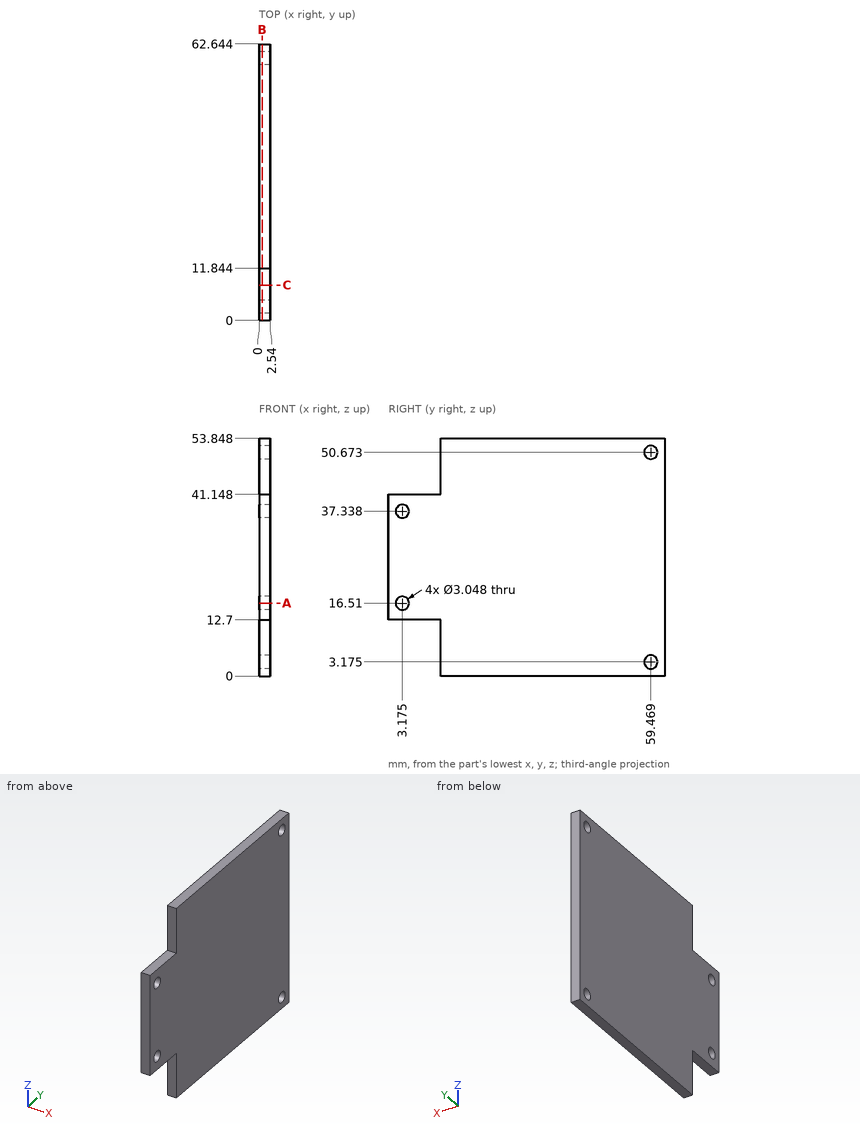
Geometry check sheet. Reference: drawing and pictorial views, mm from the part's lowest x, y, z. Coordinates: 2 decimals unless noted, no trailing zeros. Order: outer loops, then holes, each group sorted by start corner. A loop starts at its lowest first (then second) coordinate and runs counter-clockwise, first axis right, second up.
Item 1: Section check C-C (y = 8). Enter the section's corners in (x, z).
Item 2: Section check B-B (x = 0.65). Enter the section's corners in (y, z) (1 decimal).
Item 3: Section check A-A (z = 16.51). Enter the section's corners in (x, y), plus the area to 3 significant figures.
Item 4: Scan lines: line 1 along Y through (x, z) = (0.6, 50.5) (1 decimal); line 2 along Y through (x, z) = (1.1, 42.5); line 3 along Y through (x, z) = (0.3, 17.5). Record each from-to range of solid material in increasing order.
Item 5: Depth check by flat-ended pin: pin 1 (1.3 mm diameter, centred on x = 1, y = 8, fed in from -Z); pin 2 (0.8 mm diameter, centred on x = 1.5, y = 4, fed in from +Z). Enter the tip coordinate at first touch or a pass-through.
Check sheet entries:
1. outline: (0, 12.7) - (2.54, 12.7) - (2.54, 41.15) - (0, 41.15) - close
2. outline: (0, 12.7) - (11.8, 12.7) - (11.8, 0) - (62.6, 0) - (62.6, 53.8) - (11.8, 53.8) - (11.8, 41.1) - (0, 41.1) - close; hole circle Ø3 at (3.2, 16.5); hole circle Ø3 at (3.2, 37.3); hole circle Ø3 at (59.5, 3.2); hole circle Ø3 at (59.5, 50.7)
3. outline: (0, 0) - (2.54, 0) - (2.54, 1.65) - (0, 1.65) - close; (0, 4.7) - (2.54, 4.7) - (2.54, 62.64) - (0, 62.64) - close
3. area: 151 mm2
4. line 1: y = 11.8 to 58, 61 to 62.6
4. line 2: y = 11.84 to 62.64
4. line 3: y = 0 to 2.02, 4.33 to 62.64
5. pin 1: stops at z = 12.7
5. pin 2: stops at z = 41.15
